Source: CAD feature listing. Evaluate the final solid. Frame: model axes, mm. A direction names the side the tool comes from. Give positions to 0.01 mm unless a question says otherwise; leave off trailing zeros. Loops run counter-clockwise (first coordinate to the right, second up) from the corner with the lowest first, then second, coordinate; pieces in that order, holes last. Notation, with made-up numbers: M -32.5,22 L 21.5,22 A19 ccw 21.5,41 Z; hole C 28.5,-32.75 d8. An arc over 180 degrees is marked long. Put each result on its own line as item: value. Start each with the question number.
```python
from build123d import *

# Parameters (mm, degrees)
SKETCH_3_R      = 2
SKETCH_3_W      = 6
SKETCH_3_H      = 2
EXTRUDE_1_DEPTH = 1.5


with BuildPart() as part:
    # 草图3 → 凸台-拉伸1 (new, symmetric)
    with BuildSketch(Plane.XY):
        with BuildLine():
            Line((0, 5), (43.909830056, 5))
            ThreePointArc((43.909830056, 5), (49.5, 7.5), (55.090169944, 5))
            Line((55.090169944, 5), (162, 5))
            ThreePointArc((162, 5), (167, 0), (162, -5))
            Line((162, -5), (55.090169944, -5))
            ThreePointArc((55.090169944, -5), (49.5, -7.5), (43.909830056, -5))
            Line((43.909830056, -5), (0, -5))
            ThreePointArc((0, -5), (-5, 0), (0, 5))
        make_face()
        with Locations((162, 0)):
            Circle(SKETCH_3_R, mode=Mode.SUBTRACT)
        Circle(SKETCH_3_R, mode=Mode.SUBTRACT)
        with Locations((49.5, 0)):
            Circle(SKETCH_3_R, mode=Mode.SUBTRACT)
        with Locations((72.5, 0)):
            Rectangle(SKETCH_3_W, SKETCH_3_H, mode=Mode.SUBTRACT)
        with Locations((132.5, 0)):
            Rectangle(SKETCH_3_W, SKETCH_3_H, mode=Mode.SUBTRACT)
    extrude(amount=EXTRUDE_1_DEPTH, both=True)


solid = part.part
```
1. Contact query for flat-ended pins moving along their axis: pin 1 (0.9 mm diameter, centred on x = 133.5, z = 0.5, fed in from -Y); pin 2 (1.5 mm diameter, centred on x = 94, z = -0.5, fed in from +Y). Output: stop coordinate, or through.
2. Pull-direction query (X, two-part tool) for faces 1 (the face through (47.502, 0.088, -0.021)), 2 (the face through (82, 0, -1.5)), 3 (the face through (49.6, -7.5, 0)); classes: released by +X, released by -X, zero draft, split by the parting line, or undercut.
3. Set-up query: faces 4 (the face through (108, 5, 0)), 5 (the face through (22, 5, 0)), 6 (the face through (72, -1, 0)). Return all of +Z, -Z, +X, -X, +Y, -Y with unobstructed straight access to the full face (end or side cutting, diameter ignored); none if empty.
4. Section A-A, the plane x = 49.5. Output: boundary loops of the cut face in (y, z), plus the area to 3 significant figures.
5. Section D-D, the plane x = 8.5. Output: boundary loops of the cut face in (y, z), plus the area to 3 significant figures.
6. Section B-B, the plane z = 0.35. Output: boundary loops of the cut face in (x, y).
7. Ray query, line 1 (Y direction, x = 49.5, z = -0.45); line 2 (Y direction, x = 162, z = 0.3); line 3 (X direction, y = 1.5, z = -0.95). Return the intervals inside material, ascending.
8. Section C-C, the plane x = 73. Output: boundary loops of the cut face in (y, z).
Results found:
1. pin 1: y = -5
1. pin 2: y = 5
2. face 1: undercut
2. face 2: zero draft
2. face 3: split by the parting line
3. face 4: +Z, -Z, +X, +Y
3. face 5: +Z, -Z, -X, +Y
3. face 6: +Z, -Z
4. outline: M -7.5,-1.5 L -2,-1.5 L -2,1.5 L -7.5,1.5 Z; M 2,-1.5 L 7.5,-1.5 L 7.5,1.5 L 2,1.5 Z
4. area: 33.0 mm²
5. outline: M -5,-1.5 L 5,-1.5 L 5,1.5 L -5,1.5 Z
5. area: 30.0 mm²
6. outline: M 0,-5 L 43.91,-5 A7.5 ccw 55.09,-5 L 162,-5 A5 ccw 162,5 L 55.09,5 A7.5 ccw 43.91,5 L 0,5 A5 ccw Z; hole C 0,0 d4; hole C 49.5,0 d4; hole M 69.5,-1 L 75.5,-1 L 75.5,1 L 69.5,1 Z; hole M 129.5,-1 L 135.5,-1 L 135.5,1 L 129.5,1 Z; hole C 162,0 d4
7. line 1: -7.5 to -2, 2 to 7.5
7. line 2: -5 to -2, 2 to 5
7. line 3: -4.77 to -1.32, 1.32 to 48.18, 50.82 to 160.68, 163.32 to 166.77
8. outline: M -5,-1.5 L -1,-1.5 L -1,1.5 L -5,1.5 Z; M 1,-1.5 L 5,-1.5 L 5,1.5 L 1,1.5 Z
